Geometry check sheet. Reference: drawing and pictorial views, mm from the part's lowest x, y, z. A direction names the side the tool comes from. Give positions to 0.01 mm unless a question says otherwise; leave off trailing zeros. Order: outer loops, then holes, each group sorted by start corner. A loop starts at its lowest first (then second) coordinate and runs counter-clockwise, first axis right, second up.
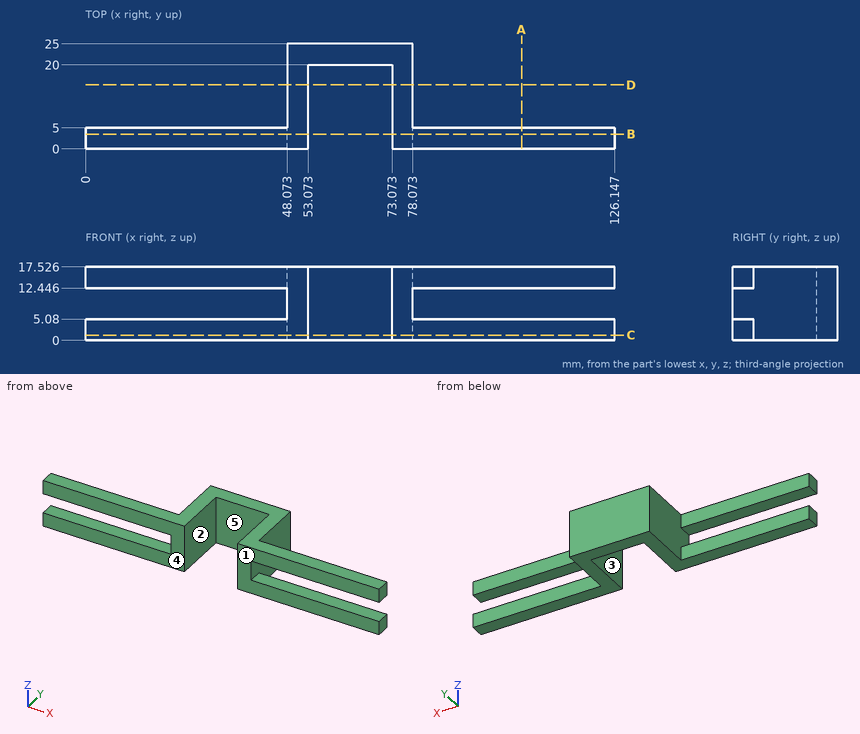
(1) Cross-section at C-C on z = 1.25. Enter the section's corners in (x, y).
Response values:
outline: (0, 0) - (53.07, 0) - (53.07, 20) - (73.07, 20) - (73.07, 0) - (126.15, 0) - (126.15, 5) - (78.07, 5) - (78.07, 25) - (48.07, 25) - (48.07, 5) - (0, 5) - close
(2) Gauge pin test, flat ends, axial feed: pin 1 Ø10 at (x, y) = (64.5, 4) entering from -Z; pin 2 Ø5.5 at (y, z) = (18, 12) entering from -X; pin 3 Ø9 at (y, z) = (14, 10.5) entering from +X; pin 4 Ø1.5 at (x, z) = (35, 2) entering from +Y. Record the tip position at first contact, or that the pin passes through.
Response values:
pin 1: passes through
pin 2: stops at x = 48.07
pin 3: stops at x = 78.07
pin 4: stops at y = 5
(3) Cross-section at A-A on x = 104. Enter the section's corners in (y, z), then the cut area to 3 significant figures.
Response values:
outline: (0, 0) - (5, 0) - (5, 5.08) - (0, 5.08) - close; (0, 12.45) - (5, 12.45) - (5, 17.53) - (0, 17.53) - close
area: 50.8 mm2
(4) Cross-section at B-B on y = 3.5. Enter the section's corners in (x, z), then the cut area to 3 significant figures.
Response values:
outline: (0, 0) - (53.07, 0) - (53.07, 17.53) - (0, 17.53) - (0, 12.45) - (48.07, 12.45) - (48.07, 5.08) - (0, 5.08) - close; (73.07, 0) - (126.15, 0) - (126.15, 5.08) - (78.07, 5.08) - (78.07, 12.45) - (126.15, 12.45) - (126.15, 17.53) - (73.07, 17.53) - close
area: 1,150 mm2
(5) Cross-section at D-D on y = 15.25. Enter the section's corners in (x, z), then the cut area to 3 significant figures.
Response values:
outline: (48.07, 0) - (53.07, 0) - (53.07, 17.53) - (48.07, 17.53) - close; (73.07, 0) - (78.07, 0) - (78.07, 17.53) - (73.07, 17.53) - close
area: 175 mm2
(6) Release check for a two-part mould opening along X. For the marked faces 1, 2 and 3 record: released by +X, released by -X, zero draft, split by the parting line, or undercut.
Response values:
face 1: zero draft
face 2: undercut
face 3: undercut
(7) Material ranges on L1, parallel to X at y = 15.5, z = 1.5; L2, parallel to Y at x = 58.5, z = 8.75; L3, parallel to Y at x = 87, z = 16.25, recorded low to high.
Response values:
L1: x = 48.07 to 53.07, 73.07 to 78.07
L2: y = 20 to 25
L3: y = 0 to 5
(8) Set-up check for the marked faces 4 and 5: record each of +Z, -Z, +X, -X, +Y, -Y from which the full face is reachable in a straight line by a thin tool's end or side.
Response values:
face 4: +Z, -Z, +X, -X, -Y
face 5: +Z, -Z, -Y
